from build123d import *

# Parameters (mm, degrees)
CUT_EXTRUDE1_DEPTH = 3.175
CHAMFER1_SIZE      = 0.5334


with BuildPart() as part:
    # Sketch1 → Revolve1 (revolve)
    with BuildSketch(Plane(origin=(0, 0, 0), x_dir=(1, 0, 0), z_dir=(0, 1, 0)), mode=Mode.PRIVATE) as revolve1_sk:
        with BuildLine():
            Line((0, 0), (0, -25.4))
            Line((0, -25.4), (3.96875, -25.4))
            Line((3.96875, -25.4), (3.96875, 0))
            Line((3.96875, 0), (6.9469, 0))
            Line((6.9469, 0), (6.9469, 0.7874))
            ThreePointArc((6.9469, 0.7874), (5.294601142, 2.758916257), (3.175, 4.2164))
            Line((3.175, 4.2164), (0, 4.2164))
            Line((0, 4.2164), (0, 0))
        make_face()
    revolve(revolve1_sk.sketch.rotate(Axis((0, 0, 0), (0, 0, 1)), 180), axis=Axis((0, 0, 0), (0, 0, 1)))

    # Sketch2 → Cut-Extrude1 (cut)
    with BuildSketch(Plane(origin=(0, 0, -4.2164), x_dir=(-1, 0, 0), z_dir=(0, 0, -1))):
        Polygon((2.749630657, 0), (1.374815329, 2.38125), (-1.374815329, 2.38125), (-2.749630657, 0), (-1.374815329, -2.38125), (1.374815329, -2.38125), align=None)
    extrude(amount=-CUT_EXTRUDE1_DEPTH, mode=Mode.SUBTRACT)

    # Chamfer1
    chamfer1_edges = [part.edges().sort_by_distance(p)[0] for p in [
        (3.96875, 0, 25.4),
    ]]
    chamfer(chamfer1_edges, length=CHAMFER1_SIZE)


solid = part.part
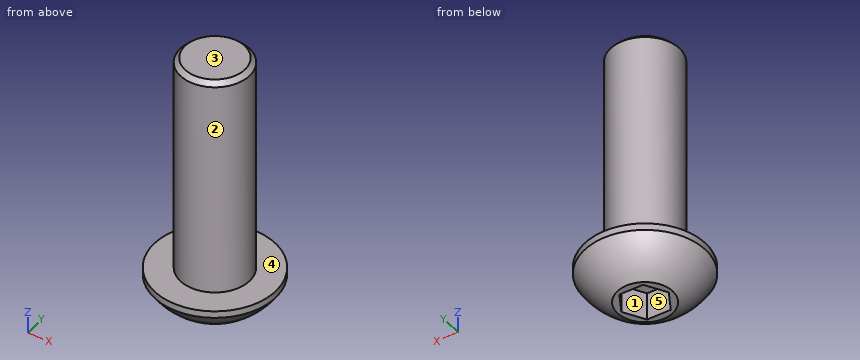
Build history of the part. All positions in model axes, mm. Face numbers are marked on the shaded views. A direction names the side the tool comes from. Round coordinates to 2 decimals unless told otherwise and drop trailing zeros. Write each loop counter-clockwise with the first axis right and the second up, starting at its lowest first coordinate (ties: lowest second). Pieces come first, ordered by that corner, then holes. Notation, with made-up numbers: M 37.25,-20 L 75.25,-20 A18 cw 75.25,-9 Z; hole C -13,64 d10. An arc over 180 degrees is marked long. Use CSV: the item, a comma, the result in double quotes.
1. Saw through at A-A (z = 23.25). Give the cut face in (x, y).
Reply:
outline,"C 0,0 d7.94"
2. Wall check: probe 1 along Z at (x, y) = (1, 1.5); probe 2 along Y at (x, z) = (0, 10.25); probe 3 along Z at (x, y) = (6, 0.5). Give the ranges that are in metal, low to high. Write a range as from..to.
Reply:
probe 1,"z = -1.04..25.4"
probe 2,"y = -3.97..3.97"
probe 3,"z = -2.02..0"
3. Two-plate mould, pull along Y, no slides. Class the marked faces 1, 2 and 3: +Y half, -Y half, draft (parallel to the pull), parting line (faces both ways), or undercut.
Reply:
face 1,"undercut"
face 2,"parting line"
face 3,"draft"
4. Flat gauge pins, fed straight in: pin 1 (2.5 mm diameter, centred on x = 0.5, y = 0, fed in from -Z); pin 2 (4 mm diameter, centred on x = -3, z = 21, fed in from +Y); pin 3 (4 mm diameter, centred on x = 0.5, z = 4, fed in from +Y). Where does each tip first touch, or does it go through?
Reply:
pin 1,"stops at z = -1.04"
pin 2,"stops at y = 3.84"
pin 3,"stops at y = 3.97"
5. Tool access for the marked faces 4 and 5: list every direction of +Z, -Z, +X, -X, +Y, -Y with a clear straight run to the whole face (end or side of a thin tool).
Reply:
face 4,"+Z"
face 5,"-Z"
